The model under review builds one solid part; all positions refer to its coordinate system, in mm. A direction names the side the tool comes from. Coordinates: 2 decimals unless noted, no trailing zeros. Order: outer loops, then holes, each group sorted by start corner. A loop starts at its lowest first (then second) coordinate and runs counter-clockwise, first axis right, second up. Notation, with made-up numbers: (0, -37) -> (42, -37) arc R18 ccw to (42, -28) -> close; hole circle Ø1 at (31, -1.75). An arc over 180 degrees is marked (long way). Use one line per item in the form item = value.
from build123d import *

# Parameters (mm, degrees)
SKETCH1_W           = 60
SKETCH1_H           = 90
SKETCH1_R           = 0.9
SKETCH1_R_2         = 1.55
SKETCH1_W_2         = 12.5
SKETCH1_H_2         = 22.5
BOSS_EXTRUDE1_DEPTH = 5
SKETCH2_W           = 20
SKETCH2_H           = 20
BOSS_EXTRUDE2_DEPTH = 20
FILLET1_R           = 10
SKETCH3_R           = 6
CUT_EXTRUDE1_DEPTH  = 99.107084352
CUT_EXTRUDE2_REACH  = 59.663
SKETCH5_W           = 60
SKETCH5_H           = 5
BOSS_EXTRUDE3_DEPTH = 51
CUT_EXTRUDE3_REACH  = 104.548
SKETCH7_W           = 19
SKETCH7_H           = 5
BOSS_EXTRUDE4_DEPTH = 10


with BuildPart() as part:
    # Sketch1 → Boss-Extrude1 (new body)
    with BuildSketch(Plane.XY):
        Rectangle(SKETCH1_W, SKETCH1_H)
        with Locations((-3, -33.25)):
            Circle(SKETCH1_R, mode=Mode.SUBTRACT)
        with Locations((-3, -6.75)):
            Circle(SKETCH1_R, mode=Mode.SUBTRACT)
        with Locations((8, -38)):
            Circle(SKETCH1_R_2, mode=Mode.SUBTRACT)
        with Locations((8, -2)):
            Circle(SKETCH1_R_2, mode=Mode.SUBTRACT)
        with Locations((-3, -20)):
            Rectangle(SKETCH1_W_2, SKETCH1_H_2, mode=Mode.SUBTRACT)
    extrude(amount=BOSS_EXTRUDE1_DEPTH)

    # Sketch2 → Boss-Extrude2 (add)
    with BuildSketch(Plane.XY.offset(5)):
        with Locations((-20, -35)):
            Rectangle(SKETCH2_W, SKETCH2_H)
        with Locations((-20, 35)):
            Rectangle(SKETCH2_W, SKETCH2_H)
        with Locations((20, 35)):
            Rectangle(SKETCH2_W, SKETCH2_H)
        with Locations((20, -35)):
            Rectangle(SKETCH2_W, SKETCH2_H)
    extrude(amount=BOSS_EXTRUDE2_DEPTH)

    # Fillet1
    fillet1_edges = [part.edges().sort_by_distance(p)[0] for p in [
        (10, -35, 25),
        (30, -35, 25),
        (30, 35, 25),
        (10, 35, 25),
        (-30, 35, 25),
        (-10, 35, 25),
        (-10, -35, 25),
        (-30, -35, 25),
    ]]
    fillet(fillet1_edges, radius=FILLET1_R - 0.0001)  # a hair under: the kernel refuses the full size

    # Sketch3 → Cut-Extrude1 (cut, through all)
    with BuildSketch(Plane.XZ.offset(45)):
        with Locations(Location((-20, 15, 0), (0, 0, 270))):
            Circle(SKETCH3_R)
        with Locations(Location((20, 15, 0), (0, 0, 270))):
            Circle(SKETCH3_R)
    extrude(amount=-CUT_EXTRUDE1_DEPTH, mode=Mode.SUBTRACT)

    # Sketch4 → Cut-Extrude2 (cut, up to next)
    with BuildSketch(Plane.XY.offset(5), mode=Mode.PRIVATE) as cut_extrude2_sk1:
        with BuildLine():
            Line((-30, 25), (-30, -25))
            ThreePointArc((-30, -25), (-15.845240526, 0), (-30, 25))
        make_face()
    cut_extrude2_tool1 = extrude(cut_extrude2_sk1.sketch, amount=-CUT_EXTRUDE2_REACH, mode=Mode.PRIVATE) & part.part
    # Sketch4 → Cut-Extrude2 (cut, up to next)
    with BuildSketch(Plane.XY.offset(5), mode=Mode.PRIVATE) as cut_extrude2_sk2:
        with BuildLine():
            Line((30, 25), (30, -25))
            ThreePointArc((30, -25), (15.845240526, 0), (30, 25))
        make_face()
    cut_extrude2_tool2 = extrude(cut_extrude2_sk2.sketch, amount=-CUT_EXTRUDE2_REACH, mode=Mode.PRIVATE) & part.part
    add(cut_extrude2_tool1.solids().sort_by_distance((-24.20079, 0, 5))[0], mode=Mode.SUBTRACT)
    add(cut_extrude2_tool2.solids().sort_by_distance((24.20079, 0, 5))[0], mode=Mode.SUBTRACT)

    # Sketch5 → Boss-Extrude3 (add)
    with BuildSketch(Plane(origin=(0, 45, 0), x_dir=(1, 0, 0), z_dir=(0, 1, 0))):
        with Locations((0, -2.5)):
            Rectangle(SKETCH5_W, SKETCH5_H)
    extrude(amount=BOSS_EXTRUDE3_DEPTH)

    # Sketch6 → Cut-Extrude3 (cut, up to next)
    with BuildSketch(Plane.XY.offset(5), mode=Mode.PRIVATE) as cut_extrude3_sk1:
        with BuildLine():
            Line((-9.5, 91), (-9.5, 96))
            Line((-9.5, 96), (-30, 96))
            Line((-30, 96), (-30, 45))
            ThreePointArc((-30, 45), (-14.856951526, 65.819402311), (-9.5, 91))
        make_face()
    cut_extrude3_tool1 = extrude(cut_extrude3_sk1.sketch, amount=-CUT_EXTRUDE3_REACH, mode=Mode.PRIVATE) & part.part
    # Sketch6 → Cut-Extrude3 (cut, up to next)
    with BuildSketch(Plane.XY.offset(5), mode=Mode.PRIVATE) as cut_extrude3_sk2:
        with BuildLine():
            Line((9.5, 91), (9.5, 96))
            Line((9.5, 96), (30, 96))
            Line((30, 96), (30, 45))
            ThreePointArc((30, 45), (14.856951526, 65.819402311), (9.5, 91))
        make_face()
    cut_extrude3_tool2 = extrude(cut_extrude3_sk2.sketch, amount=-CUT_EXTRUDE3_REACH, mode=Mode.PRIVATE) & part.part
    add(cut_extrude3_tool1.solids().sort_by_distance((-21.41045, 76.034299, 5))[0], mode=Mode.SUBTRACT)
    add(cut_extrude3_tool2.solids().sort_by_distance((21.41045, 76.034299, 5))[0], mode=Mode.SUBTRACT)

    # Sketch7 → Boss-Extrude4 (add)
    with BuildSketch(Plane.XY.offset(5)):
        with Locations((0, 93.5)):
            Rectangle(SKETCH7_W, SKETCH7_H)
    extrude(amount=BOSS_EXTRUDE4_DEPTH)


solid = part.part
Item 1: We need section D-D (x = -5.5). Write out the cut boundary in (y, z), plus the area to 4 significant figures.
Results found:
outline = (-45, 0) -> (-31.25, 0) -> (-31.25, 5) -> (-45, 5) -> close; (-8.75, 0) -> (96, 0) -> (96, 15) -> (91, 15) -> (91, 5) -> (-8.75, 5) -> close
area = 642.5 mm²
Item 2: Clearance check with flat-ended pins moving along their axes: pin 1 (6 mm diameter, centred on x = 7, y = -6.5, fed in from +Z); pin 2 (4 mm diameter, centred on y = -17.5, z = 1.5, fed in from +X); pin 3 (1.5 mm diameter, centred on y = 93, z = 6, fed in from -X). State where each tip first meets the part, or that it passes through.
Results found:
pin_1 = 5
pin_2 = 23.33
pin_3 = -9.5
Item 3: Draft analysis for pull direction Z (two halves, no side actions). For faces 6 (the face through (0, 25, 0)), 7 (the face through (-18.198, 34.86, 9.277)), 8 (the face through (15.85, -0.42, 2.54)), state which applies: released by +Z, released by -Z, zero draft, split by the parting line, or undercut.
Results found:
face_6 = released by -Z
face_7 = undercut
face_8 = zero draft
Item 4: Tool access review of faces 1 (the face through (-9.25, -20, 2)), 2 (the face through (13.01, 35.14, 22.15)), 3 (the face through (-16, 25, 10)), 4 (the face through (-16, 45, 10)), 5 (the face through (-9.5, 93, 7)): name each direction out of +Z, -Z, +X, -X, +Y, -Y from which nothing blocks a thin tool from reaching the whole face with its end or side.
Results found:
face_1 = +Z, -Z
face_2 = +Z, +Y, -Y
face_3 = +Z, +X, -X
face_4 = +Z, +X, -X, +Y
face_5 = +Z, -Z, -X, +Y
Item 5: We need section A-A (y = -38). State how many separate pieces and enclosed holes the cut face has, plus the area to 3 significant figures.
Results found:
separate_pieces = 2
enclosed_holes = 2
area = 772 mm²
Item 6: We need section C-C (z = 2.25). Write out the cut boundary in (x, y).
Results found:
outline = (-30, -45) -> (30, -45) -> (30, -25) arc R29.15 cw to (30, 25) -> (30, 45) arc R61.86 cw to (9.5, 91) -> (9.5, 96) -> (-9.5, 96) -> (-9.5, 91) arc R61.86 cw to (-30, 45) -> (-30, 25) arc R29.15 cw to (-30, -25) -> close; hole (-9.25, -31.25) -> (3.25, -31.25) -> (3.25, -8.75) -> (-9.25, -8.75) -> close; hole circle Ø1.8 at (-3, -33.25); hole circle Ø1.8 at (-3, -6.75); hole circle Ø3.1 at (8, -38); hole circle Ø3.1 at (8, -2)
Item 7: To check wall thickness, follow L1, parallel to Y at x = 8, z = 1.2; L2, parallel to Y at x = -3, z = 1.9; L3, parallel to X at y = 43.5, z = 14.75. State the ranges of each line that lie inside material, in increasing order. Write a range as from..to.
Results found:
L1 = -45..-39.55, -36.45..-3.55, -0.45..96
L2 = -45..-34.15, -32.35..-31.25, -8.75..-7.65, -5.85..96
L3 = -30..-25.99, -14.01..-10, 10..14.01, 25.99..30
Item 8: We need section B-B (x = 8). Write out the cut boundary in (y, z), plus the area to 3 significant figures.
Results found:
outline = (-45, 0) -> (-39.55, 0) -> (-39.55, 5) -> (-45, 5) -> close; (-36.45, 0) -> (-3.55, 0) -> (-3.55, 5) -> (-36.45, 5) -> close; (-0.45, 0) -> (96, 0) -> (96, 15) -> (91, 15) -> (91, 5) -> (-0.45, 5) -> close
area = 724 mm²
